from build123d import *

# Parameters (mm, degrees)
SKETCH1_W           = 100
SKETCH1_H           = 60
BOSS_EXTRUDE1_DEPTH = 30
CUT_EXTRUDE1_DEPTH  = 20


with BuildPart() as part:
    # Sketch1 → Boss-Extrude1 (new, symmetric)
    with BuildSketch(Plane(origin=(0, 0, 0), x_dir=(0, 0, -1), z_dir=(1, 0, 0))):
        with Locations((-50, 0)):
            Rectangle(SKETCH1_W, SKETCH1_H)
    extrude(amount=BOSS_EXTRUDE1_DEPTH, both=True)

    # Sketch2 → Cut-Extrude1 (cut, symmetric)
    with BuildSketch(Plane(origin=(0, 0, 0), x_dir=(0, 0, -1), z_dir=(1, 0, 0))):
        with BuildLine():
            Line((0, 15), (0, -15))
            add(Edge.make_bspline(
                [(0, -15), (-25, -15), (-25, -10), (-50, -10)],
                knots=[0, 0, 0, 0, 1, 1, 1, 1], degree=3))
            Line((-50, -10), (-50, 20))
            add(Edge.make_bspline(
                [(0, 15), (-25, 15), (-25, 20), (-50, 20)],
                knots=[0, 0, 0, 0, 1, 1, 1, 1], degree=3))
        make_face()
    cut_extrude1 = extrude(amount=CUT_EXTRUDE1_DEPTH, both=True, mode=Mode.SUBTRACT)

    # Mirror1: Cut-Extrude1 across plane
    add(cut_extrude1.mirror(Plane(origin=(-20, 20, 50), x_dir=(1, 0, 0), z_dir=(0, 0, 1))), mode=Mode.SUBTRACT)


solid = part.part
Could you check a few things on this model? Use its own coordinates, in mm. Give positions to 0.01 mm unless a question says otherwise; leave off trailing zeros. Order: outer loops, then holes, each group sorted by start corner. A loop starts at its lowest first (then second) coordinate and runs counter-clockwise, first axis right, second up.
1. I need wall thicknesses on L1, parallel to X at y = -4.5, z = 44; L2, parallel to Y at x = 17.5, z = 52; L3, parallel to Y at x = -8, z = 90. Which ranges of each line are inside material? Lowest first, please.
2. Suppose I cut it at A-A (y = -6.5). List the corners of the cut face in (x, z) for me.
3. We'd pull the mould along X, two halves only. Please class faces 1 (the flat face through (20, 3, 51)), 2 (the flat face through (0, 30, 51)), 3 (the flat face through (30, 0, 51)), 4 (the flat face through (-30, 0, 51)): pulls with the +X half, pulls with the -X half, needs draft (parallel to the pull), parting line crosses it, or undercut.
Solved:
1. L1: x = -30 to -20, 20 to 30
1. L2: y = -30 to -10.01, 19.99 to 30
1. L3: y = -30 to -14.68, 15.32 to 30
2. outline: (-30, 0) - (-20, 0) - (-20, 100) - (-30, 100) - close; (20, 0) - (30, 0) - (30, 100) - (20, 100) - close
3. face 1: undercut
3. face 2: needs draft
3. face 3: pulls with the +X half
3. face 4: pulls with the -X half
